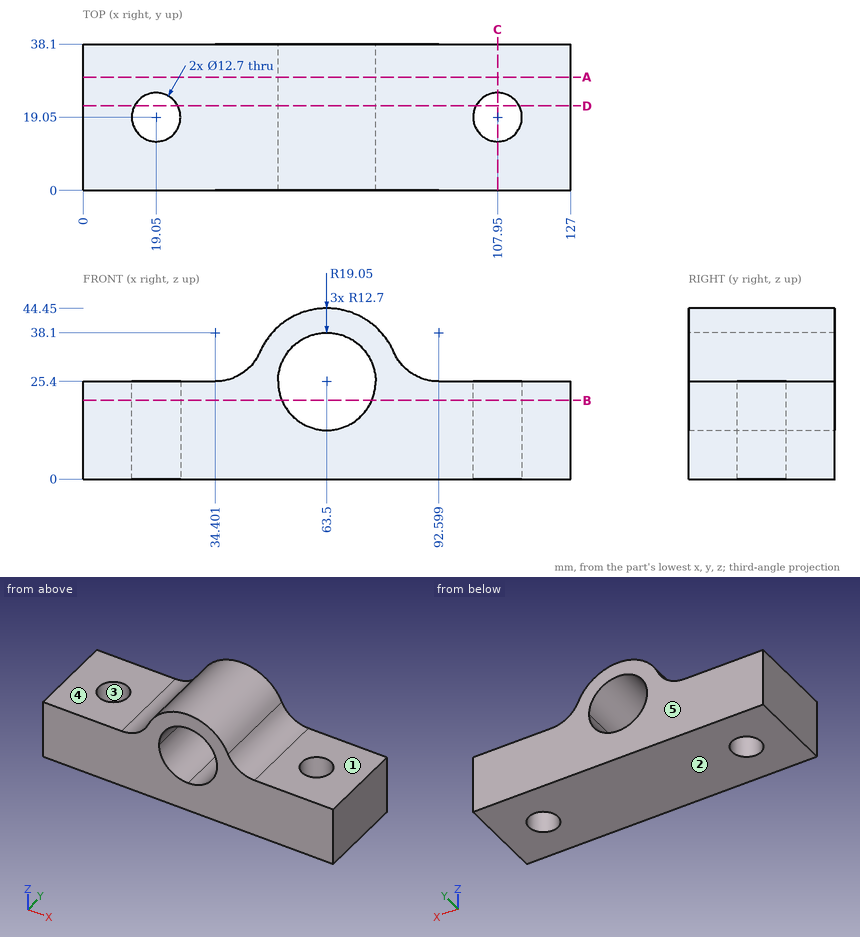
Verification items for this drawing (mm, ordinates from the low corner). A direction names the side the tool comes from. Round coordinates to 2 decimals unless told otherwise and drop trailing zeros. Write each loop counter-clockwise with the first axis right and the second up, starting at its lowest first coordinate (ties: lowest second). Pieces come first, ordered by that corner, then holes. Notation, with made-up numbers: (57, 80) - (98, 80) arc R27 cw to (98, 114) - close; hole circle Ø4 at (-30, 53.25). An arc over 180 degrees is marked (long way). Answer as a JSON object with one key per item and string values. Group by question number.
Q1. Thickness scan on line 1 (Y direction, x = 107.95, z = 6.75); line 2 (X direction, y = 14, z = 19.5) (1 decimal); line 3 (X direction, y = 19.5, z = 19) (1 decimal). Record the ranges inside material, lowest first.
Q2. Mould release check, pull along Y, two halves, no side actions. Record for the marked faces 3, 4 and 5: released by +Y, released by -Y, zero draft, split by the parting line, or undercut.
Q3. Tool access check on the marked faces 1 and 2. Record the directions out of +Z, -Z, +X, -X, +Y, -Y that give a thin tool (end or side, any length) a straight path to the whole face; none if there is none.
Q4. Go/stop test with flat-tipped pins: pin 1 Ø16.5 at (x, y) = (107.95, 19.05) entering from +Z; pin 2 Ø10 at (x, y) = (19.05, 19.05) entering from +Z; pin 3 Ø1 at (y, z) = (11.5, 38) entering from -X; pin 4 Ø2 at (x, y) = (65.5, 21) entering from +Z. Record where each tip stops, or that it passes through.
Q5. Section check D-D, the plane y = 22. Enter the section's corners in (x, z), plus the area to 3 significant figures.
Q6. Section check B-B, the plane z = 20.5. Enter the section's corners in (x, y), plus the area to 3 significant figures.
Q7. Section check A-A, the plane y = 29.5. Enter the section's corners in (x, z).
Q8. Section check C-C, the plane x = 107.95. Enter the section's corners in (y, z), plus the area to 3 significant figures.
Found:
{
 "1": {"line 1": "y = 0 to 12.7, 25.4 to 38.1", "line 2": "x = 0 to 15.2, 22.9 to 52.3, 74.7 to 104.1, 111.8 to 127", "line 3": "x = 0 to 12.7, 25.4 to 52.5, 74.5 to 101.6, 114.3 to 127"},
 "2": {"face 3": "undercut", "face 4": "zero draft", "face 5": "released by +Y"},
 "3": {"face 1": "+Z, +X, +Y, -Y", "face 2": "-Z, +X, -X, +Y, -Y"},
 "4": {"pin 1": "stops at z = 25.4", "pin 2": "passes through", "pin 3": "stops at x = 48.79", "pin 4": "stops at z = 44.42"},
 "5": {"outline": "(0, 0) - (13.43, 0) - (13.43, 25.4) - (0, 25.4) - close; (24.67, 0) - (102.33, 0) - (102.33, 25.4) - (92.6, 25.4) arc R12.7 cw to (80.96, 33.02) arc R19.05 ccw to (46.04, 33.02) arc R12.7 cw to (34.4, 25.4) - (24.67, 25.4) - close; (113.57, 0) - (127, 0) - (127, 25.4) - (113.57, 25.4) - close; hole circle Ø25.4 at (63.5, 25.4)", "area": "2,750 mm^2"},
 "6": {"outline": "(0, 0) - (51.78, 0) - (51.78, 38.1) - (0, 38.1) - close; (75.22, 0) - (127, 0) - (127, 38.1) - (75.22, 38.1) - close; hole circle Ø12.7 at (19.05, 19.05); hole circle Ø12.7 at (107.95, 19.05)", "area": "3,690 mm^2"},
 "7": {"outline": "(0, 0) - (127, 0) - (127, 25.4) - (92.6, 25.4) arc R12.7 cw to (80.96, 33.02) arc R19.05 ccw to (46.04, 33.02) arc R12.7 cw to (34.4, 25.4) - (0, 25.4) - close; hole circle Ø25.4 at (63.5, 25.4)"},
 "8": {"outline": "(0, 0) - (12.7, 0) - (12.7, 25.4) - (0, 25.4) - close; (25.4, 0) - (38.1, 0) - (38.1, 25.4) - (25.4, 25.4) - close", "area": "645 mm^2"}
}
